Read the model definition and answer for the solid it produces. Units are mm, in the model's axes. A direction names the side the tool comes from. Round coordinates to 2 decimals unless told otherwise and drop trailing zeros. Order: outer loops, then holes, each group sorted by start corner. A loop starts at its lowest first (then second) coordinate and runs counter-clockwise, first axis right, second up. Notation, with made-up numbers: (-9, 72) -> (25, 72) arc R10 cw to (25, 83) -> close; hole circle Ø8 at (-39, -22). An arc over 180 degrees is marked (long way). One line per item, written item: value. Start each with the question number.
1. The mould has two halves that part along X. Classify faces 1 (the face through (0, 3, -12.7)), 2 (the face through (5.278, 0, 125)), 3 (the face through (0, 5.278, 125)), 4 (the face through (-5.278, 0, 125)): released by +X, released by -X, zero draft, split by the parting line, or undercut.
2. Flat-ended cylindrical pins translate along their axes: pin 1 Ø1.5 at (x, z) = (3, 144) entering from +Y; pin 2 Ø6 at (x, z) = (0.5, 142.5) entering from +Y; pin 3 Ø1.6 at (x, z) = (0, 96.5) entering from -Y; pin 4 Ø3 at (x, y) = (-1, 5.5) entering from -Z. Find the tip coordinate at first contact, or state that the pin passes through.
3. Consider line 1 (Y direction, x = 10.25, z = 76); line 2 (X direction, y = 6.75, z = 15.5); line 3 (X direction, y = -7.5, z = 169.5). Determine where each line is inside the solid, lowest interval first.
4. For faces 5 (the face through (0, -5.278, 125)), 6 (the face through (0, 3, 266.7)), determine the directions among +Z, -Z, +X, -X, +Y, -Y from which every point of the face is accessible in a straight line to the end or side of a thin tool.
5. Section A-A (x = 0) is taken. Give the vertices of the cut face in (y, z).
Autodesk Inventor part; units mm, degrees
ref_plane "Start Plane" through (0, 0, -12.7) normal (0, 0, 1) x (1, 0, 0)
ref_plane "End Plane" through (0, 0, 266.7) normal (0, 0, 1) x (1, 0, 0)
ref_plane "Work Plane4" through (10.6172, 0, 266.7) normal (0, 0, 1) x (1, 0, 0)
ref_plane "Start Plane" through (0, 0, -12.7) normal (0, 0, 1) x (1, 0, 0)
ref_plane "End Plane" through (0, 0, 266.7) normal (0, 0, 1) x (1, 0, 0)
sketch "Sketch" plane through (0, 0, 0) normal (0, 0, 1) x (1, 0, 0)
  arc A0 (-11.6332, 12.7) -> (-12.7, 11.6332) centre (-11.6332, 11.6332) ccw
  arc A1 (-5.3594, 10.5664) -> (-5.3594, 12.7) centre (-5.3594, 11.6332) ccw
  arc A2 (-12.7, 5.3594) -> (-10.5664, 5.3594) centre (-11.6332, 5.3594) ccw
  line L0 (-10.5664, 7.493) -> (-10.5664, 5.3594)
  line L1 (-7.493, 10.5664) -> (-5.3594, 10.5664)
  arc A3 (-9.6992, 7.8522) -> (-10.5664, 7.493) centre (-10.0584, 7.493) ccw
  arc A4 (-7.493, 10.5664) -> (-7.8522, 9.6992) centre (-7.493, 10.0584) ccw
  line L2 (-11.6332, 11.6332) -> (0, 0) construction
  line L3 (-5.8003, 3.9533) -> (-9.6992, 7.8522)
  line L4 (-7.8522, 9.6992) -> (-3.9533, 5.8003)
  arc A5 (-3.9533, 5.8003) -> (-2.6924, 5.278) centre (-2.6924, 7.0612) ccw
  arc A6 (-5.278, 2.6924) -> (-5.8003, 3.9533) centre (-7.0612, 2.6924) ccw
  arc A7 (0, 2.54) -> (-2.54, 0) centre (0, 0) ccw construction
  line L5 (0, 0) -> (-12.7, 0) construction
  line L6 (0, 12.7) -> (0, 0) construction
  arc A8 (-11.6332, 12.7) -> (-10.6172, 12.7) centre (-11.1252, 12.7) ccw
  arc A9 (-7.5692, 12.7) -> (-6.5532, 12.7) centre (-7.0612, 12.7) ccw
  arc A10 (-12.7, 10.6172) -> (-12.7, 11.6332) centre (-12.7, 11.1252) ccw
  arc A11 (-12.7, 6.5532) -> (-12.7, 7.5692) centre (-12.7, 7.0612) ccw
  line L7 (-12.7, 10.6172) -> (-12.7, 7.5692)
  line L8 (-12.7, 6.5532) -> (-12.7, 5.3594)
  line L9 (-10.6172, 12.7) -> (-7.5692, 12.7)
  line L10 (-6.5532, 12.7) -> (-5.3594, 12.7)
  circle A12 centre (0, 0) radius 2.54
  arc A13 (-12.7, -11.6332) -> (-11.6332, -12.7) centre (-11.6332, -11.6332) ccw
  line L11 (-12.7, -10.6172) -> (-12.7, -7.5692)
  arc A14 (-10.5664, -7.493) -> (-9.6992, -7.8522) centre (-10.0584, -7.493) ccw
  line L12 (-9.6992, -7.8522) -> (-5.8003, -3.9533)
  line L13 (-11.6332, -11.6332) -> (0, 0) construction
  line L14 (-3.9533, -5.8003) -> (-7.8522, -9.6992)
  arc A15 (-7.8522, -9.6992) -> (-7.493, -10.5664) centre (-7.493, -10.0584) ccw
  line L15 (-10.6172, -12.7) -> (-7.5692, -12.7)
  line L16 (-7.493, -10.5664) -> (-5.3594, -10.5664)
  arc A16 (-6.5532, -12.7) -> (-7.5692, -12.7) centre (-7.0612, -12.7) ccw
  line L17 (-6.5532, -12.7) -> (-5.3594, -12.7)
  arc A17 (-5.3594, -12.7) -> (-5.3594, -10.5664) centre (-5.3594, -11.6332) ccw
  arc A18 (-10.6172, -12.7) -> (-11.6332, -12.7) centre (-11.1252, -12.7) ccw
  arc A19 (-12.7, -11.6332) -> (-12.7, -10.6172) centre (-12.7, -11.1252) ccw
  arc A20 (-2.6924, -5.278) -> (-3.9533, -5.8003) centre (-2.6924, -7.0612) ccw
  arc A21 (-5.8003, -3.9533) -> (-5.278, -2.6924) centre (-7.0612, -2.6924) ccw
  line L18 (-10.5664, -7.493) -> (-10.5664, -5.3594)
  line L19 (-12.7, -6.5532) -> (-12.7, -5.3594)
  arc A22 (-10.5664, -5.3594) -> (-12.7, -5.3594) centre (-11.6332, -5.3594) ccw
  arc A23 (-12.7, -7.5692) -> (-12.7, -6.5532) centre (-12.7, -7.0612) ccw
  arc A24 (11.6332, -12.7) -> (12.7, -11.6332) centre (11.6332, -11.6332) ccw
  line L20 (10.6172, -12.7) -> (7.5692, -12.7)
  arc A25 (7.493, -10.5664) -> (7.8522, -9.6992) centre (7.493, -10.0584) ccw
  line L21 (7.8522, -9.6992) -> (3.9533, -5.8003)
  line L22 (11.6332, -11.6332) -> (0, 0) construction
  line L23 (5.8003, -3.9533) -> (9.6992, -7.8522)
  arc A26 (9.6992, -7.8522) -> (10.5664, -7.493) centre (10.0584, -7.493) ccw
  line L24 (12.7, -10.6172) -> (12.7, -7.5692)
  line L25 (10.5664, -7.493) -> (10.5664, -5.3594)
  arc A27 (12.7, -6.5532) -> (12.7, -7.5692) centre (12.7, -7.0612) ccw
  line L26 (12.7, -6.5532) -> (12.7, -5.3594)
  arc A28 (12.7, -5.3594) -> (10.5664, -5.3594) centre (11.6332, -5.3594) ccw
  arc A29 (12.7, -10.6172) -> (12.7, -11.6332) centre (12.7, -11.1252) ccw
  arc A30 (11.6332, -12.7) -> (10.6172, -12.7) centre (11.1252, -12.7) ccw
  arc A31 (5.278, -2.6924) -> (5.8003, -3.9533) centre (7.0612, -2.6924) ccw
  arc A32 (3.9533, -5.8003) -> (2.6924, -5.278) centre (2.6924, -7.0612) ccw
  line L27 (7.493, -10.5664) -> (5.3594, -10.5664)
  line L28 (6.5532, -12.7) -> (5.3594, -12.7)
  arc A33 (5.3594, -10.5664) -> (5.3594, -12.7) centre (5.3594, -11.6332) ccw
  arc A34 (7.5692, -12.7) -> (6.5532, -12.7) centre (7.0612, -12.7) ccw
  arc A35 (12.7, 11.6332) -> (11.6332, 12.7) centre (11.6332, 11.6332) ccw
  line L29 (12.7, 10.6172) -> (12.7, 7.5692)
  arc A36 (10.5664, 7.493) -> (9.6992, 7.8522) centre (10.0584, 7.493) ccw
  line L30 (9.6992, 7.8522) -> (5.8003, 3.9533)
  line L31 (11.6332, 11.6332) -> (0, 0) construction
  line L32 (3.9533, 5.8003) -> (7.8522, 9.6992)
  arc A37 (7.8522, 9.6992) -> (7.493, 10.5664) centre (7.493, 10.0584) ccw
  line L33 (10.6172, 12.7) -> (7.5692, 12.7)
  line L34 (7.493, 10.5664) -> (5.3594, 10.5664)
  arc A38 (6.5532, 12.7) -> (7.5692, 12.7) centre (7.0612, 12.7) ccw
  line L35 (6.5532, 12.7) -> (5.3594, 12.7)
  arc A39 (5.3594, 12.7) -> (5.3594, 10.5664) centre (5.3594, 11.6332) ccw
  arc A40 (10.6172, 12.7) -> (11.6332, 12.7) centre (11.1252, 12.7) ccw
  arc A41 (12.7, 11.6332) -> (12.7, 10.6172) centre (12.7, 11.1252) ccw
  arc A42 (2.6924, 5.278) -> (3.9533, 5.8003) centre (2.6924, 7.0612) ccw
  arc A43 (5.8003, 3.9533) -> (5.278, 2.6924) centre (7.0612, 2.6924) ccw
  line L36 (10.5664, 7.493) -> (10.5664, 5.3594)
  line L37 (12.7, 6.5532) -> (12.7, 5.3594)
  arc A44 (10.5664, 5.3594) -> (12.7, 5.3594) centre (11.6332, 5.3594) ccw
  arc A45 (12.7, 7.5692) -> (12.7, 6.5532) centre (12.7, 7.0612) ccw
  line L38 (-2.6924, 5.278) -> (2.6924, 5.278)
  line L39 (-5.278, 2.6924) -> (-5.278, -2.6924)
  line L40 (-2.6924, -5.278) -> (2.6924, -5.278)
  line L41 (5.278, -2.6924) -> (5.278, 2.6924)
  point P0 (0, 0)
  point P1 (0, 0)
  dimension "d2" = 2.1336
  dimension "d3" = 6.2738
  dimension "d4" = 6.2738
  dimension "d5" = 1.0668
  dimension "d6" = 2.1336
  dimension "d7" = 2.1336
  dimension "d8" = 1.016
  dimension "d9" = 1.016
  dimension "d10" = 135
  dimension "d11" = 2.667
  dimension "d12" = 4.572
  dimension "d13" = 4.572
  dimension "d14" = 2.667
  dimension "d15" = 5.08
  dimension "d16" = 45
  dimension "d19" = 45
  dimension "d20" = 0.508
  dimension "d21" = 4.572
  dimension "d22" = 1.016
  dimension "d23" = 4.572
  dimension "d24" = 1.016
  dimension "d25" = 0.508
  dimension "d26" = 0.508
  dimension "d27" = 0.508
  dimension "d28" = 12.7
  dimension "d37" = 360
  dimension "d47" = 10.5664
  dimension "d48" = 12.7
extrude "Body" add sketch "Sketch" along normal up to surface (279.4 mm away) from surface at -12.7
sketch "Sketch2" plane through (0, 0, 0) normal (0, 0, 1) x (1, 0, 0)
  line L0 (0, 0) -> (10, 0)
ref_plane "Work Plane3" through (0, 0, 0) normal (0, -1, 0) x (1, 0, 0)
sketch "Sketch3" plane through (0, 0, 0) normal (0, -1, 0) x (1, 0, 0)
  line L0 (-2, -12.7) -> (12, -12.7)
  line L1 (-2, 266.7) -> (12, 266.7)
  dimension "d60" = 279.4
ref_plane "Work Plane4" through (10.6172, 0, 266.7) normal (0, 0, 1) x (1, 0, 0)
split "Split1" plane through (10.6172, 0, 266.7) removes the side toward (0, 0, 1)
ref_plane "Work Plane5" through (0, -7.5692, -12.7) normal (0, 0, -1) x (-1, 0, 0)
split "Split2" plane through (0, -7.5692, -12.7) removes the side toward (0, 0, -1)
ref_plane "Work Plane6" through (-10.6172, -279.4, -12.7) normal (0, 0, -1) x (-1, 0, 0)
split "Split3" plane through (-10.6172, -279.4, -12.7) removes the side toward (0, 0, -1)
equation "\"d3\" = d4"
equation "\"d6\" = d7"
equation "\"d11\" = d14"
equation "\"d12\" = d13"
equation "\"d23\" = d21"
equation "\"d24\" = d30"
equation "\"d26\" = 0.5 * d24"
equation "\"d27\" = 0.5 * d22"
equation "\"Width\" = 2 * d28"
equation "\"Height\" = 2 * d48"
equation "\"G_OFFSET_START\" = 12.7"
equation "\"G_OFFSET_END\" = -12.7"
equation "\"d55\" = -G_OFFSET_START"
equation "\"d56\" = Length + G_OFFSET_END"
equation "\"G_L\" = 279.4"
properties part number "1010_80_20" material "Aluminum-6061"
Answer:
1. face 1: zero draft
1. face 2: released by +X
1. face 3: undercut
1. face 4: released by -X
2. pin 1: y = 5.63
2. pin 2: y = 5.47
2. pin 3: y = -5.28
2. pin 4: z = -12.7
3. line 1: -12.7 to -7.96, 7.96 to 12.7
3. line 2: -12.3 to -10.57, -8.6 to -4.9, 4.9 to 8.6, 10.57 to 12.3
3. line 3: -12.44 to -10.57, -9.35 to -5.65, 5.65 to 9.35, 10.57 to 12.44
4. face 5: +Z, -Z, -Y
4. face 6: +Z, +X, -X, +Y, -Y
5. outline: (-5.28, -12.7) -> (-2.54, -12.7) -> (-2.54, 266.7) -> (-5.28, 266.7) -> close; (2.54, -12.7) -> (5.28, -12.7) -> (5.28, 266.7) -> (2.54, 266.7) -> close
